Part model, mm, in its own coordinate system. Round coordinates to 2 decimals unless told otherwise and drop trailing zeros. Loops run counter-clockwise (first coordinate to the right, second up) from the corner with the lowest first, then second, coordinate; pieces in that order, holes last. Notation, with made-up numbers: (58.25, -40) -> (96.25, -40) arc R24 ccw to (96.25, -8) -> close; hole circle Ø2 at (8, 63.5). An arc over 180 degrees is marked (long way). Answer as CSV lines item,"result".
from build123d import *

# Parameters (mm, degrees)
EXTRUDE_1_DEPTH     = 1
SKETCH_2_W          = 5
SKETCH_2_H          = 30
CUT_EXTRUDE_1_DEPTH = 10
CHAMFER_1_SIZE      = 10
CHAMFER_1_SIZE_2    = 7.071067812
CHAMFER_2_SIZE      = 10
SKETCH_3_R          = 1.6
CUT_EXTRUDE_2_DEPTH = 10
SKETCH_4_W          = 20
SKETCH_4_H          = 75.961940777
EXTRUDE_2_DEPTH     = 1
CHAMFER_3_SIZE      = 10


with BuildPart() as part:
    # 草图1 → 凸台-拉伸1 (new body)
    with BuildSketch(Plane(origin=(0, 0, 0), x_dir=(1, 0, 0), z_dir=(0, 1, 0))):
        Polygon((0, 0), (53.033008589, 0), (53.033008589, 55), (0, 108.033008589), align=None)
    extrude(amount=EXTRUDE_1_DEPTH)

    # 草图2 → 切除-拉伸1 (cut)
    with BuildSketch(Plane.XZ):
        with Locations((2.5, -15)):
            Rectangle(SKETCH_2_W, SKETCH_2_H)
    extrude(amount=-CUT_EXTRUDE_1_DEPTH, mode=Mode.SUBTRACT)

    # 倒角1
    # the kernel refuses this chamfer: 10, 7.071067812 mm, written as the material it adds along each edge
    with BuildSketch(Plane(origin=(5, 0, -30), x_dir=(0.027495876610586403, 0, 0.9996219169112968), z_dir=(0, 1, 0))) as chamfer_1_piece_1_section:
        Polygon((CHAMFER_1_SIZE * 0.999621916911, -CHAMFER_1_SIZE * 0.0274958766106), (-CHAMFER_1_SIZE * 0.0274958766106, -CHAMFER_1_SIZE * 0.999621916911), (0, 0), align=None)
    chamfer_1_piece_1 = extrude(amount=1, mode=Mode.PRIVATE)
    chamfer_1_piece_1 = split(chamfer_1_piece_1, bisect_by=Plane(origin=(0, 0.5, -26.065989159), z_dir=(1, 0, 0)), keep=Keep.TOP, mode=Mode.PRIVATE)
    add(chamfer_1_piece_1)
    # the kernel refuses this chamfer: 10, 7.071067812 mm, written as the material it takes off along each edge
    with BuildSketch(Plane(origin=(0, -25.71682988, -108.033008589), x_dir=(-0.056478249472490825, 0, 0.9984038297885897), z_dir=(0, 1, 0))) as chamfer_1_2_piece_1:
        Polygon((CHAMFER_1_SIZE_2 * 0.99840382977, CHAMFER_1_SIZE_2 * 0.0564782494714), (CHAMFER_1_SIZE * 0.666041965215, CHAMFER_1_SIZE * 0.745914271598), (0, 0), align=None)
    extrude(amount=52.433659759, mode=Mode.SUBTRACT)
    with BuildSketch(Plane(origin=(5, -25.71682988, 0), x_dir=(0.9996219169112968, 0, 0.027495876610586372), z_dir=(0, 1, 0))) as chamfer_1_2_piece_2:
        Polygon((CHAMFER_1_SIZE * 0.999621916911, CHAMFER_1_SIZE * 0.0274958766106), (-CHAMFER_1_SIZE * 0.0274958766106, CHAMFER_1_SIZE * 0.999621916911), (0, 0), align=None)
    extrude(amount=52.433659759, mode=Mode.SUBTRACT)
    with BuildSketch(Plane(origin=(53.033008589, -25.71682988, 0), x_dir=(-0.9996219169112968, 0, 0.027495876610586372), z_dir=(0, 1, 0))) as chamfer_1_2_piece_3:
        Polygon((CHAMFER_1_SIZE * 0.999621916911, -CHAMFER_1_SIZE * 0.0274958766106), (-CHAMFER_1_SIZE * 0.0274958766106, -CHAMFER_1_SIZE * 0.999621916911), (0, 0), align=None)
    extrude(amount=52.433659759, mode=Mode.SUBTRACT)

    # 倒角2
    chamfer_2_edges = [part.edges().sort_by_distance(p)[0] for p in [
        (53.033008589, 0.5, -55),
    ]]
    chamfer(chamfer_2_edges, length=CHAMFER_2_SIZE)

    # 草图3 → 切除-拉伸2 (cut)
    with BuildSketch(Plane.XZ):
        with Locations(Location((22.980970389, -77.980970389, 0), (0, 0, 270))):
            Circle(SKETCH_3_R)
        with Locations(Location((48.033008589, -27.5, 0), (0, 0, 270))):
            Circle(SKETCH_3_R)
        with Locations(Location((29.016504294, -5, 0), (0, 0, 270))):
            Circle(SKETCH_3_R)
    extrude(amount=-CUT_EXTRUDE_2_DEPTH, mode=Mode.SUBTRACT)

    # 草图4 → 凸台-拉伸2 (add)
    with BuildSketch(Plane.XZ):
        with Locations((-10, -62.980970389)):
            Rectangle(SKETCH_4_W, SKETCH_4_H)
    extrude(amount=-EXTRUDE_2_DEPTH)

    # 倒角3
    chamfer_3_edges = [part.edges().sort_by_distance(p)[0] for p in [
        (-20, 0.5, -25),
        (-20, 0.5, -100.961940777),
    ]]
    chamfer(chamfer_3_edges, length=CHAMFER_3_SIZE)


solid = part.part
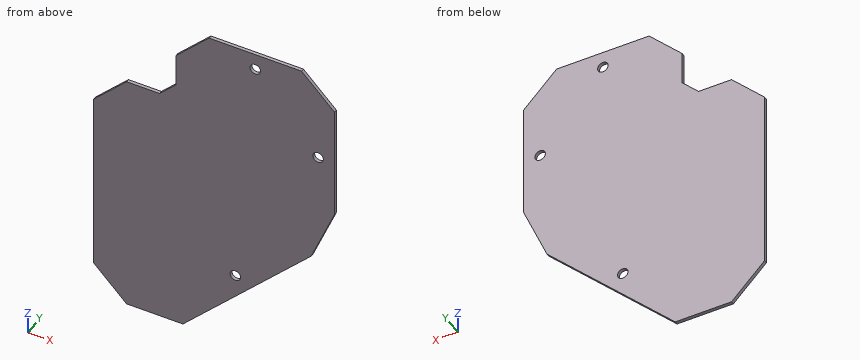
Q1. Saw through at D-D, the plane x = -13. Write the cut outline in (y, z), then the cut area to 3 significant figures.
Geometry results:
outline,"(0, -97.96) -> (1, -97.96) -> (1, -28) -> (0, -28) -> close"
area,"70.0 mm2"
Q2. Drill centre lines: line 1 along Z through (x, y) = (23.5, 0.1); line 2 along Z through (x, y) = (22.5, 0.6); line 3 along Z through (x, y) = (-5, 0.8). Where is each one in solid material? Low to high.
Geometry results:
line 1,"-84.53 to -79.49, -76.47 to 0"
line 2,"-85.53 to -79.51, -76.45 to 0"
line 3,"-100.96 to -25"
Q3. Saw through at C-C, the plane z = -5. Write the cut outline in (x, y), then the cut area to 3 significant figures.
Geometry results:
outline,"(10, 0) -> (27.42, 0) -> (27.42, 1) -> (10, 1) -> close; (30.62, 0) -> (48.03, 0) -> (48.03, 1) -> (30.62, 1) -> close"
area,"34.8 mm2"
Q4. Saw through at A-A, the plane z = -27.5. Write the cut outline in (x, y), then the cut area to 3 significant figures.
Geometry results:
outline,"(-12.5, 0) -> (46.43, 0) -> (46.43, 1) -> (-12.5, 1) -> close; (49.63, 0) -> (53.03, 0) -> (53.03, 1) -> (49.63, 1) -> close"
area,"62.3 mm2"
Q5. Saw through at B-B, the plane y = 0.25. Write the cut outline in (x, z), then the cut area to 3 significant figures.
Geometry results:
outline,"(-20, -90.96) -> (-10, -100.96) -> (7.07, -100.96) -> (45.96, -62.07) -> (53.03, -45) -> (53.03, -10) -> (43.03, 0) -> (15, 0) -> (5, -10) -> (5, -20) -> (0, -25) -> (-10, -25) -> (-20, -35) -> close; hole circle Ø3.2 at (22.98, -77.98); hole circle Ø3.2 at (29.02, -5); hole circle Ø3.2 at (48.03, -27.5)"
area,"5,450 mm2"
Q6. Drop a flat-ended pin along its axis: P1, Ø3, axis at x = 48.03, z = -27.5, coming from the -Y side. Give the stop position or say it passes through.
Geometry results:
P1,"through"
